Geometry: final body of the model. Coordinates: model frame, mm. Face numbers are marked on the shaded views. A direction names the side the tool comes from. Give positions to 0.01 mm unless a question says otherwise; leave off trailing zeros. Loops run counter-clockwise (first coordinate to the right, second up) from the corner with the lowest first, then second, coordinate; pieces in that order, holes last. Notation, with made-up numbers: (-4, 43.5) - (1, 43.5) arc R29 cw to (1, 63.5) - close; hole circle Ø1 at (61.25, -8). An arc over 180 degrees is marked (long way). Answer in a Markdown table with one row per item.
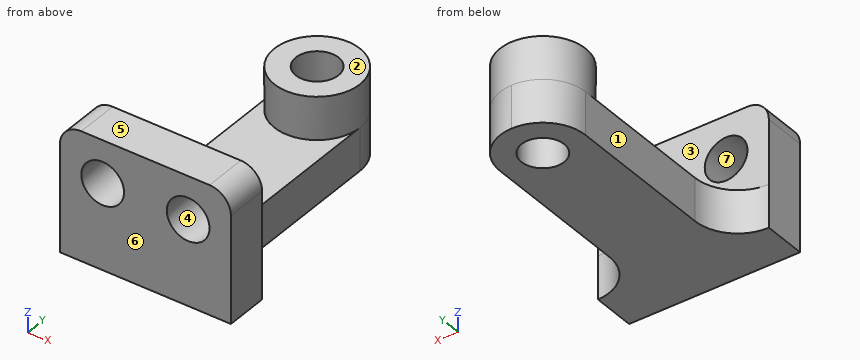
Autodesk Inventor part; units mm, degrees
ref_plane "YZ Plane" through (0, 0, 0) normal (1, 0, 0) x (0, 1, 0)
ref_plane "XZ Plane" through (0, 0, 0) normal (0, 1, 0) x (-1, 0, 0)
ref_plane "XY Plane" through (0, 0, 0) normal (0, 0, 1) x (1, 0, 0)
sketch "Sketch1" plane through (0, 0, 0) normal (0, 0, 1) x (1, 0, 0)
  line L0 (-3.9739, 11.3944) -> (46.8261, 11.3944)
  line L1 (46.8261, 11.3944) -> (46.8261, -71.1556)
  line L2 (46.8261, -71.1556) -> (-3.9739, -71.1556)
  line L3 (-3.9739, -71.1556) -> (-3.9739, 11.3944)
  point P0 (0, 0)
  dimension "d0" = 50.8
  dimension "d1" = 82.55
extrude "Extrusion1" add sketch "Sketch1" along normal blind 38.1
sketch "Sketch2" plane through (46.8261, -71.1556, 0) normal (1, 0, 0) x (0, 0, -1)
  line L0 (0, 82.55) -> (-38.1, 82.55)
  line L1 (-38.1, 82.55) -> (-12.7, 82.55)
  line L2 (-12.7, 82.55) -> (-12.7, 12.7)
  line L3 (-12.7, 12.7) -> (-38.1, 12.7)
  line L4 (-38.1, 12.7) -> (-38.1, 82.55)
  point P0 (0, 71.1556)
  dimension "d4" = 25.4
  dimension "d5" = 69.85
extrude "Extrusion2" cut sketch "Sketch2" against normal through all
sketch "Sketch3" plane through (46.8261, -58.4556, 12.7) normal (0, 0, 1) x (1, 0, 0)
  line L0 (-50.8, 69.85) -> (0, 69.85)
  line L1 (-50.8, 69.85) -> (-38.1, 69.85)
  line L2 (-38.1, 69.85) -> (-38.1, 0)
  line L3 (-38.1, 0) -> (-50.8, 0)
  line L4 (-50.8, 0) -> (-50.8, 69.85)
  line L5 (0, 69.85) -> (-12.7, 69.85)
  line L6 (-12.7, 69.85) -> (-12.7, 0)
  line L7 (-12.7, 0) -> (0, 0)
  line L8 (0, 0) -> (0, 69.85)
  point P0 (-46.8261, 58.4556)
  dimension "d8" = 12.7
  dimension "d9" = 69.85
  dimension "d10" = 12.7
  dimension "d11" = 69.85
extrude "Extrusion3" cut sketch "Sketch3" against normal through all
sketch "Sketch4" plane through (8.7261, -58.4556, 12.7) normal (0, 0, 1) x (1, 0, 0)
  line L0 (0, 69.85) -> (0, 0) construction
  line L1 (25.4, 0) -> (0, 0) construction
  line L2 (25.4, 0) -> (25.4, 69.85) construction
  line L3 (0, 69.85) -> (25.4, 69.85) construction
  circle A0 centre (12.7, 57.15) radius 12.7
  circle A1 centre (12.7, 57.15) radius 6.35
  point P0 (-8.7261, 58.4556)
  dimension "d14" = 12.7
extrude "Extrusion4" add sketch "Sketch4" along normal mid plane 25.4
sketch "Sketch5" plane through (8.7261, 11.3944, 12.7) normal (0, 0, 1) x (1, 0, 0)
  arc A0 (12.7, 0) -> (0, -12.7) centre (12.7, -12.7) ccw
  line L0 (0, 0) -> (12.7, 0)
  line L1 (0, 0) -> (0, -12.7)
  arc A1 (25.4, -12.7) -> (12.7, 0) centre (12.7, -12.7) ccw
  line L2 (25.4, -12.7) -> (25.4, 0)
  line L3 (12.7, 0) -> (25.4, 0)
  point P0 (-8.7261, -11.3944)
extrude "Extrusion5" cut sketch "Sketch5" against normal through all
sketch "Sketch6" plane through (21.4261, -1.3056, 12.7) normal (0, 0, 1) x (1, 0, 0)
  circle A0 centre (0, 0) radius 6.35
  point P0 (-21.4261, 1.3056)
extrude "Extrusion6" cut sketch "Sketch6" against normal through all
sketch "Sketch7" plane through (46.8261, -58.4556, 38.1) normal (0, 1, 0) x (1, 0, 0)
  line L0 (-50.8, 0) -> (-50.8, 38.1) construction
  line L1 (0, 0) -> (-50.8, 0) construction
  line L2 (0, 38.1) -> (0, 0) construction
  line L3 (-12.7, 38.1) -> (0, 38.1) construction
  line L4 (-12.7, 25.4) -> (-12.7, 38.1) construction
  line L5 (-12.7, 25.4) -> (-38.1, 25.4) construction
  line L6 (-38.1, 25.4) -> (-38.1, 38.1) construction
  line L7 (-50.8, 38.1) -> (-38.1, 38.1) construction
  line L8 (-50.8, 0) -> (-50.8, 38.1) construction
  line L9 (0, 0) -> (-50.8, 0) construction
  line L10 (0, 38.1) -> (0, 0) construction
  line L11 (-12.7, 38.1) -> (0, 38.1) construction
  line L12 (-12.7, 25.4) -> (-12.7, 38.1) construction
  line L13 (-12.7, 25.4) -> (-38.1, 25.4) construction
  line L14 (-38.1, 25.4) -> (-38.1, 38.1) construction
  line L15 (-50.8, 38.1) -> (-38.1, 38.1) construction
  line L16 (-38.1, 12.7) -> (-12.7, 12.7) construction
  point P0 (-46.8261, 38.1)
hole "Hole1" at (8.7261, -58.4556, 25.4) at (34.1261, -58.4556, 25.4) direction (0, -1, 0) diameter 12.7 end through all
fillet "Fillet1" radius 6.35 2 edges at (-3.9739, -64.8056, 38.1) (46.8261, -64.8056, 38.1)
fillet "Fillet2" radius 12.7 2 edges at (8.7261, -58.4556, 6.35) (34.1261, -58.4556, 6.35)
Q1. Cut plane B-B (y = -63). Output: boundary loops of the cut face in (x, z), and give its area (3 significant figures).
Check values:
| item | result |
|---|---|
| outline | (-3.97, 0) - (46.83, 0) - (46.83, 31.75) arc R6.35 ccw to (40.48, 38.1) - (2.38, 38.1) arc R6.35 ccw to (-3.97, 31.75) - close; hole circle Ø12.7 at (8.73, 25.4); hole circle Ø12.7 at (34.13, 25.4) |
| area | 1,660 mm² |
Q2. Cut plane D-D (y = -36). Output: boundary loops of the cut face in (x, z), and give its area (3 significant figures).
Check values:
| item | result |
|---|---|
| outline | (8.73, 0) - (34.13, 0) - (34.13, 12.7) - (8.73, 12.7) - close |
| area | 323 mm² |
Q3. Draft query along Z for the marked faces 5, 6 and 7. Return one class per face: pulls with the +Z half, pulls with the -Z half, needs draft (parallel to the pull), parting line crosses it, or undercut.
Check values:
| item | result |
|---|---|
| face 5 | pulls with the +Z half |
| face 6 | needs draft |
| face 7 | undercut |
Q4. First-contact query: pin 1 (3 mm diameter, centred on x = 12, z = 15, fed in from +Y); pin 2 (1.5 mm diameter, centred on y = 0, z = 5.5, fed in from -X); pin 3 (6.5 mm diameter, centred on y = -16, z = 6.5, fed in from +X); pin 4 (16.5 mm diameter, centred on x = 21.43, y = -1.31, fed in from -Z). Flat tips, straight axial feed; report the tip coordinate or a pass-through.
Check values:
| item | result |
|---|---|
| pin 1 | y = 8.62 |
| pin 2 | x = 8.74 |
| pin 3 | x = 34.13 |
| pin 4 | z = 0 |
Q5. Cut plane C-C (y = 2.5). Output: boundary loops of the cut face in (x, z), and give its area (3 significant figures).
Check values:
| item | result |
|---|---|
| outline | (9.31, 0) - (16.34, 0) - (16.34, 25.4) - (9.31, 25.4) - close; (26.51, 0) - (33.54, 0) - (33.54, 25.4) - (26.51, 25.4) - close |
| area | 357 mm² |
Q6. Reachability of the marked faces 1, 2, 3 and 4 from +Z, -Z, +X, -X, +Y, -Y: full face, straight path, thin tool, end or side. Return the list, or none.
Check values:
| item | result |
|---|---|
| face 1 | +Z, -Z, -X, +Y |
| face 2 | +Z, +X, -X, +Y |
| face 3 | +Z, +X, -X |
| face 4 | -Y |
Q7. Cut plane A-A (z = 21.5). Output: boundary loops of the cut face in (x, y), and give its area (3 significant figures).
Check values:
| item | result |
|---|---|
| outline | (-3.97, -71.16) - (3.71, -71.16) - (3.71, -58.46) - (-3.97, -58.46) - close; circle Ø25.4 at (21.43, -1.31); (13.74, -71.16) - (29.11, -71.16) - (29.11, -58.46) - (13.74, -58.46) - close; (39.14, -71.16) - (46.83, -71.16) - (46.83, -58.46) - (39.14, -58.46) - close; hole circle Ø12.7 at (21.43, -1.31) |
| area | 771 mm² |
Q8. Material intervals for line 1 along X through (y, z) = (-64.5, 25.4); line 2 along Y through (x, z) = (21.5, 4); line 3 along Z through (x, y) = (18.5, -25), sorted ascending.
Check values:
| item | result |
|---|---|
| line 1 | -3.97 to 2.38, 15.08 to 27.78, 40.48 to 46.83 |
| line 2 | -71.16 to -7.66, 5.04 to 11.39 |
| line 3 | 0 to 12.7 |
